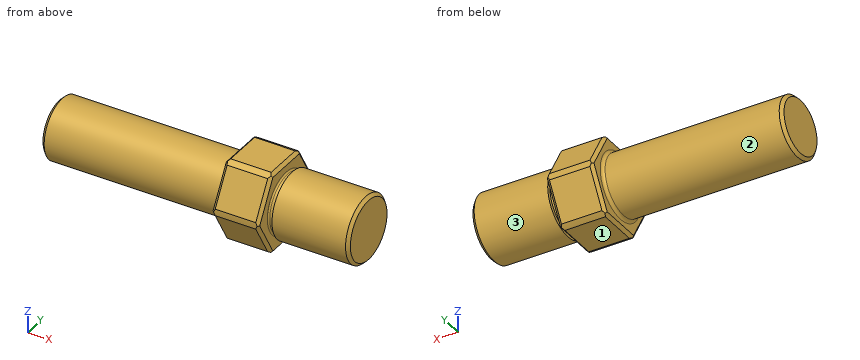
```python
from build123d import *

# Parameters (mm, degrees)
CHAFL_N1_SIZE           = 1
REDONDEO1_R             = 1
CROQUIS2_R              = 21.776851014
CORTAR_EXTRUIR1_DEPTH   = 11
CHAFL_N2_SIZE           = 1
SALIENTE_EXTRUIR1_DEPTH = 15.5
CROQUIS12_W             = 2
CROQUIS12_H             = 2
REDONDEO3_R             = 0.5
SALIENTE_EXTRUIR3_START = 10
CROQUIS15_R             = 10
SALIENTE_EXTRUIR3_DEPTH = 10
CHAFL_N6_SIZE           = 1
CHAFL_N8_SIZE           = 1
CORTAR_EXTRUIR3_START   = -15.009619
CROQUIS17_R             = 19.700918629
CROQUIS17_R_2           = 15
CORTAR_EXTRUIR3_DEPTH   = 14.519238


with BuildPart() as part:
    # Croquis1 → Revolución1 (revolve)
    with BuildSketch(Plane(origin=(0, 0, 0), x_dir=(1, 0, 0), z_dir=(0, 1, 0))):
        Polygon((0, 0), (0, 11), (-50, 11), (-54, 11), (-54, 10), (-104, 10), (-104, 0), align=None)
    revolve(axis=Axis((0, 0, 0), (-1, 0, 0)))

    # Chaflán1
    chafl_n1_edges = [part.edges().sort_by_distance(p)[0] for p in [
        (0, 0, 11),
    ]]
    chamfer(chafl_n1_edges, length=CHAFL_N1_SIZE)

    # Redondeo1
    redondeo1_edges = [part.edges().sort_by_distance(p)[0] for p in [
        (-54, 0, 10),
    ]]
    fillet(redondeo1_edges, radius=REDONDEO1_R - 0.0001)  # a hair under: the kernel refuses the full size

    # Croquis2 → Cortar-Extruir1 (cut)
    with BuildSketch(Plane(origin=(0, 0, 0), x_dir=(0, 0, -1), z_dir=(1, 0, 0))):
        Circle(CROQUIS2_R)
    extrude(amount=-CORTAR_EXTRUIR1_DEPTH, mode=Mode.SUBTRACT)

    # Chaflán2
    chafl_n2_edges = [part.edges().sort_by_distance(p)[0] for p in [
        (-11, 0, 11),
    ]]
    chamfer(chafl_n2_edges, length=CHAFL_N2_SIZE)

    # Croquis10 → Saliente-Extruir1 (add)
    with BuildSketch(Plane(origin=(-54, 0, 0), x_dir=(0, 0, -1), z_dir=(1, 0, 0))):
        Polygon((-13.5, 7.794228634), (-13.5, -7.794228634), (0, -15.588457268), (13.5, -7.794228634), (13.5, 7.794228634), (0, 15.588457268), align=None)
    extrude(amount=SALIENTE_EXTRUIR1_DEPTH)

    # Croquis12 → Cortar-Revolución1 (revolve, cut)
    with BuildSketch(Plane(origin=(0, 0, 0), x_dir=(1, 0, 0), z_dir=(0, 1, 0)), mode=Mode.PRIVATE) as cortar_revoluci_n1_sk:
        with Locations((-37.5, -10.75)):
            Rectangle(CROQUIS12_W, CROQUIS12_H)
    revolve(cortar_revoluci_n1_sk.sketch.rotate(Axis((0, 0, 0), (-1, 0, 0)), 180), axis=Axis((0, 0, 0), (-1, 0, 0)), mode=Mode.SUBTRACT)

    # Redondeo3
    redondeo3_edges = [part.edges().sort_by_distance(p)[0] for p in [
        (-38.5, 0, 9.75),
    ]]
    fillet(redondeo3_edges, radius=REDONDEO3_R)

    # Croquis15 → Saliente-Extruir3 (add)
    with BuildSketch(Plane.ZY.offset(104).offset(SALIENTE_EXTRUIR3_START)):
        Circle(CROQUIS15_R)
    extrude(amount=-SALIENTE_EXTRUIR3_DEPTH)

    # Chaflán6
    chafl_n6_edges = [part.edges().sort_by_distance(p)[0] for p in [
        (-114, 0, -10),
    ]]
    chamfer(chafl_n6_edges, length=CHAFL_N6_SIZE)

    # Chaflán8
    chafl_n8_edges = [part.edges().sort_by_distance(p)[0] for p in [
        (-54, 11.691342951, 6.75),
        (-54, 0, 13.5),
        (-54, -11.691342951, 6.75),
        (-54, -11.691342951, -6.75),
        (-54, 0, -13.5),
        (-54, 11.691342951, -6.75),
        (-38.5, 11.691342951, 6.75),
        (-38.5, 0, 13.5),
        (-38.5, -11.691342951, 6.75),
        (-38.5, -11.691342951, -6.75),
        (-38.5, 0, -13.5),
        (-38.5, 11.691342951, -6.75),
    ]]
    chamfer(chafl_n8_edges, length=CHAFL_N8_SIZE)

    # Croquis17 → Cortar-Extruir3 (cut)
    with BuildSketch(Plane.ZY.offset(54).offset(CORTAR_EXTRUIR3_START)):
        Circle(CROQUIS17_R)
        Circle(CROQUIS17_R_2, mode=Mode.SUBTRACT)
    extrude(amount=CORTAR_EXTRUIR3_DEPTH, mode=Mode.SUBTRACT)


solid = part.part
```
CAD build for the part. Positions are in the model's coordinates, mm. Face numbers are marked on the shaded views. A direction names the side the tool comes from. Round coordinates to 2 decimals unless told otherwise and drop trailing zeros. Loops run counter-clockwise (first coordinate to the right, second up) from the corner with the lowest first, then second, coordinate; pieces in that order, holes last. Notation, with made-up numbers: M 17,7 L 21,7 A7 ccw 21,18 Z; hole C -4,-17 d3. An arc over 180 degrees is marked long. Use a Markdown table: item, result. Add a question column.
(1) Which spindle directions (+Z, -Z, +X, -X, +Y, -Y) get a long thin tool onto all of the face, cutting with end or side? Do the marked faces 1, 2 and 3. Say none if no direction does.
(2) Cut at D-D (x = -34). Give the cut face in (y, z).
(3) Cut at A-A (y = 0). Give the cut face in (x, z), and give its area (3 significant figures).
(4) Drill centre lines: line 1 (X direction, y = 11, z = 1.75); line 2 (X direction, y = 10, z = 2.75); line 3 (Z direction, x = -57, y = 0). Where is each one in solid material? Low to high.
(5) Cut at B-B (x = -52). Give the cut face in (y, z), and give its area (3 significant figures).
(6) Flat gauge pins, fed straight in: pin 1 (1 mm diameter, centred on y = -9, z = 7, fed in from +X); pin 2 (3 mm diameter, centred on x = -87, z = 8, fed in from -Y); pin 3 (10 mm diameter, centred on x = -68.5, y = 8.5, fed in from +Z); pin 4 (1.5 mm diameter, centred on x = -79, y = -11.5, fed in from -Z). Where does each tip first touch, or does it go through?
(7) Cut at C-C (x = -97). Give the cut face in (y, z), and give its area (3 significant figures).
Geometry says:
| question | item | result |
|---|---|---|
| 1 | face 1 | -Z, +X, -X, +Y, -Y |
| 1 | face 2 | -X |
| 1 | face 3 | +X |
| 2 | outline | C 0,0 d22 |
| 3 | outline | M -114,-9 L -113,-10 L -55,-10 A1 cw -54,-11 L -54,-12.5 L -53,-13.5 L -39.5,-13.5 L -38.5,-12.5 L -38.5,-10.25 A0.5 cw -38,-9.75 L -36.5,-9.75 L -36.5,-11 L -12,-11 L -11,-10 L -11,10 L -12,11 L -36.5,11 L -36.5,9.75 L -38,9.75 A0.5 cw -38.5,10.25 L -38.5,12.5 L -39.5,13.5 L -53,13.5 L -54,12.5 L -54,11 A1 cw -55,10 L -113,10 L -114,9 Z |
| 3 | area | 2,220 mm² |
| 4 | line 1 | x = -54 to -38.5 |
| 4 | line 2 | x = -54.22 to -38.5, -36.5 to -11.37 |
| 4 | line 3 | z = -10 to 10 |
| 5 | outline | M -14.96,-1.09 L -8.42,-12.41 A15 ccw -6.54,-13.5 L 6.54,-13.5 A15 ccw 8.42,-12.41 L 14.96,-1.09 A15 ccw 14.96,1.09 L 8.42,12.41 A15 ccw 6.54,13.5 L -6.54,13.5 A15 ccw -8.42,12.41 L -14.96,1.09 A15 ccw Z |
| 5 | area | 628 mm² |
| 6 | pin 1 | stops at x = -11.9 |
| 6 | pin 2 | stops at y = -7.6 |
| 6 | pin 3 | stops at z = 9.37 |
| 6 | pin 4 | passes through |
| 7 | outline | C 0,0 d20 |
| 7 | area | 314 mm² |
